```python
from build123d import *

# Parameters (mm, degrees)
F1_DEPTH = 63.5
F2_T     = -2.54
F3_R     = 6.35
F4_DEPTH = 25.4


with BuildPart() as f1:
    # F0 (on Right) → F1 (new body, symmetric)
    with BuildSketch(Plane.YZ):
        with BuildLine():
            Line((9.525, 0), (-9.525, 0))
            ThreePointArc((-9.525, 0), (0, -9.525), (9.525, 0))
        make_face()
    extrude(amount=F1_DEPTH, both=True)

    # F2
    f2_openings = [f1.faces().sort_by_distance(p)[0] for p in [
        (-63.5, 0, -4.042536),
        (0, 0, 0),
        (63.5, 0, -4.042536),
    ]]
    offset(amount=F2_T, openings=f2_openings)

    # F3 (on Top) → F4 (cut)
    with BuildSketch(Plane.XY):
        with Locations((30.042015313, 0)):
            Circle(F3_R)
    extrude(amount=-F4_DEPTH, mode=Mode.SUBTRACT)


solid = f1.part
```
For this review, take the finished solid that the model builds, in its own axes (mm). Give positions to 0.01 mm unless a question says otherwise; leave off trailing zeros. Order: outer loops, then holes, each group sorted by start corner. A loop starts at its lowest first (then second) coordinate and runs counter-clockwise, first axis right, second up.
1) Take a section at B-B (z = -4.75). Give the boundary of the cut face in (x, y).
2) The part is to be moulded in two halves that separate along X. For faces 1 (the face through (0.889, -0.154, -6.983)), 2 (the face through (63.5, 0, -8)), 3 (the face through (36.1, 1.9, -6.9)), say which applies: released by +X, released by -X, zero draft, split by the parting line, or undercut.
3) Take a section at D-D (y = -5.25). Give the boundary of the cut face in (x, z).
4) Take a section at C-C (x = 21.5). Give the boundary of the cut face in (y, z) (3 decimals).
5) Take a section at A-A (y = 0). Give the boundary of the cut face in (x, z) (3 decimals), then the cut area to 3 significant figures.
6) Insertion check: pin 1 (1 mm diameter, centred on x = 43.5, y = 5.5, fed in from -Z); pin 2 (2 mm diameter, centred on x = 7.5, z = -6.5, fed in from +Y). Each pin has a flat end and moves straight along its axis. Give the tip position at first contact, or say it passes through.
7) Wall thickness on line 1 (Y direction, x = 42, z = -0.25); line 2 (X direction, y = 0, z = -7.25); line 3 (Y direction, x = 48, z = -1.5): over which ranges is each line inside the solid? List them lowest first.
Derived:
1. outline: (-63.5, -8.26) - (63.5, -8.26) - (63.5, -5.12) - (33.8, -5.12) arc R6.35 cw to (26.29, -5.12) - (-63.5, -5.12) - close; (-63.5, 5.12) - (26.29, 5.12) arc R6.35 cw to (33.8, 5.12) - (63.5, 5.12) - (63.5, 8.26) - (-63.5, 8.26) - close
2. face 1: zero draft
2. face 2: released by +X
2. face 3: undercut
3. outline: (-63.5, -7.95) - (26.47, -7.95) - (26.47, -4.61) - (-63.5, -4.61) - close; (33.61, -7.95) - (63.5, -7.95) - (63.5, -4.61) - (33.61, -4.61) - close
4. outline: (-9.525, 0) arc R9.525 ccw to (9.525, 0) - (6.985, 0) arc R6.985 cw to (-6.985, 0) - close
5. outline: (-63.5, -9.525) - (23.692, -9.525) - (23.692, -6.985) - (-63.5, -6.985) - close; (36.392, -9.525) - (63.5, -9.525) - (63.5, -6.985) - (36.392, -6.985) - close
5. area: 290 mm2
6. pin 1: stops at z = -8.11
6. pin 2: stops at y = 7.78
7. line 1: y = -9.52 to -6.98, 6.98 to 9.52
7. line 2: x = -63.5 to 23.69, 36.39 to 63.5
7. line 3: y = -9.41 to -6.82, 6.82 to 9.41
